```python
from build123d import *

# Parameters (mm, degrees)
IZIM1_R                     = 13.8
Y_KSEKLIK_EKSTR_ZYON1_DEPTH = 3
Y_KSEKLIK_EKSTR_ZYON2_DEPTH = 100
IZIM3_W                     = 77.5
IZIM3_H                     = 53.5
KES_EKSTR_ZYON1_DEPTH       = 10
IZIM4_W                     = 8.6
IZIM4_H                     = 8.6
KES_EKSTR_ZYON2_DEPTH       = 10
IZIM5_R                     = 1.6
KES_EKSTR_ZYON3_DEPTH       = 10
IZIM6_R                     = 1.6
KES_EKSTR_ZYON4_DEPTH       = 10
KES_EKSTR_ZYON5_START       = -10
IZIM7_R                     = 1.6
KES_EKSTR_ZYON5_DEPTH       = 10
KES_EKSTR_ZYON6_START       = -10
IZIM8_R                     = 1.6
KES_EKSTR_ZYON6_DEPTH       = 10


with BuildPart() as part:
    # Çizim1 → Yükseklik-Ekstrüzyon1 (new body)
    with BuildSketch(Plane(origin=(0, 0, 0), x_dir=(1, 0, 0), z_dir=(0, 1, 0))):
        with BuildLine():
            Line((50, 0), (140, 0))
            Line((140, 0), (140, 85))
            Line((140, 85), (0, 85))
            Line((0, 85), (0, 0))
            ThreePointArc((0, 0), (25, -25), (50, 0))
        make_face()
        with Locations(Location((25, 0, 0), (0, 0, 270))):
            Circle(IZIM1_R, mode=Mode.SUBTRACT)
    extrude(amount=Y_KSEKLIK_EKSTR_ZYON1_DEPTH)

    # Çizim2 → Yükseklik-Ekstrüzyon2 (add)
    with BuildSketch(Plane(origin=(0, 3, 0), x_dir=(1, 0, 0), z_dir=(0, 1, 0))):
        with BuildLine():
            Line((140, 85), (0, 85))
            Line((0, 85), (0, 0))
            ThreePointArc((0, 0), (25, -25), (50, 0))
            Line((50, 0), (140, 0))
            Line((140, 0), (140, 85))
        make_face()
        with BuildLine():
            Line((3, 0), (3, 3))
            Line((3, 3), (3, 82))
            Line((3, 82), (137, 82))
            Line((137, 82), (137, 3))
            Line((137, 3), (47, 3))
            Line((47, 3), (47, 0))
            ThreePointArc((47, 0), (25, -22), (3, 0))
        make_face(mode=Mode.SUBTRACT)
    extrude(amount=Y_KSEKLIK_EKSTR_ZYON2_DEPTH)

    # Çizim3 → Kes-Ekstrüzyon1 (cut)
    with BuildSketch(Plane.XY):
        with Locations((95, 66.25)):
            Rectangle(IZIM3_W, IZIM3_H)
    extrude(amount=-KES_EKSTR_ZYON1_DEPTH, mode=Mode.SUBTRACT)

    # Çizim4 → Kes-Ekstrüzyon2 (cut)
    with BuildSketch(Plane.XY):
        with Locations((95, 19.062)):
            Rectangle(IZIM4_W, IZIM4_H)
    extrude(amount=-KES_EKSTR_ZYON2_DEPTH, mode=Mode.SUBTRACT)

    # Çizim5 → Kes-Ekstrüzyon3 (cut)
    with BuildSketch(Plane.XY):
        with Locations((65, 98)):
            Circle(IZIM5_R)
        with Locations((125, 98)):
            Circle(IZIM5_R)
    extrude(amount=-KES_EKSTR_ZYON3_DEPTH, mode=Mode.SUBTRACT)

    # Çizim6 → Kes-Ekstrüzyon4 (cut)
    with BuildSketch(Plane(origin=(140, 0, 0), x_dir=(0, 0, -1), z_dir=(1, 0, 0))):
        with Locations((15, 98)):
            Circle(IZIM6_R)
        with Locations((70, 98)):
            Circle(IZIM6_R)
    extrude(amount=-KES_EKSTR_ZYON4_DEPTH, mode=Mode.SUBTRACT)

    # Çizim7 → Kes-Ekstrüzyon5 (cut)
    with BuildSketch(Plane(origin=(0, 0, -85), x_dir=(-1, 0, 0), z_dir=(0, 0, -1)).offset(KES_EKSTR_ZYON5_START)):
        with Locations(Location((-125, 98, 0), (0, 0, 180))):
            Circle(IZIM7_R)
        with Locations((-15, 98)):
            Circle(IZIM7_R)
    extrude(amount=KES_EKSTR_ZYON5_DEPTH, mode=Mode.SUBTRACT)

    # Çizim8 → Kes-Ekstrüzyon6 (cut)
    with BuildSketch(Plane.ZY.offset(KES_EKSTR_ZYON6_START)):
        with Locations(Location((-70, 98, 0), (0, 0, 180))):
            Circle(IZIM8_R)
        with Locations(Location((-15, 98, 0), (0, 0, 180))):
            Circle(IZIM8_R)
    extrude(amount=KES_EKSTR_ZYON6_DEPTH, mode=Mode.SUBTRACT)


solid = part.part
```
Work out the finished part from the listing and answer in its coordinate system (mm). A direction names the side the tool comes from. Give positions to 0.01 mm unless a question says otherwise; leave off trailing zeros. Loops run counter-clockwise (first coordinate to the right, second up) from the corner with the lowest first, then second, coordinate; pieces in that order, holes last. Notation, with made-up numbers: (-9.5, -39.75) - (22.5, -39.75) arc R31 cw to (22.5, -10.75) - close; hole circle Ø8 at (38, 57.5). An arc over 180 degrees is marked (long way). One line per question, with ' | ' between items.
(1) Straight lines are drawn through the part: probe 1 along Y at (x, z) = (125, -0.8); probe 2 along Z at (x, y) = (138, 98); probe 3 along X at (y, z) = (98, -83.45). For each, find the intervals that lie inside material, in ascending order.
Recorded:
probe 1: y = 0 to 39.5, 93 to 96.4, 99.6 to 103 | probe 2: z = -85 to -71.6, -68.4 to -16.6, -13.4 to 0 | probe 3: x = 0 to 13.4, 16.6 to 123.4, 126.6 to 140
(2) The part is cut by section C-C (y = 84). Write down the section's boundary in (x, z).
Recorded:
outline: (0, -85) - (140, -85) - (140, 0) - (133.75, 0) - (133.75, -3) - (137, -3) - (137, -82) - (3, -82) - (3, 0) arc R22 cw to (47, 0) - (47, -3) - (56.25, -3) - (56.25, 0) - (50, 0) arc R25 ccw to (0, 0) - close
(3) The part is cut by section D-D (z = -41.5). Write down the section's boundary in (x, y).
Recorded:
outline: (0, 0) - (140, 0) - (140, 103) - (137, 103) - (137, 3) - (3, 3) - (3, 103) - (0, 103) - close
(4) The part is cut by section A-A (x = 76.5). Write down the section's boundary in (y, z).
Recorded:
outline: (0, -85) - (103, -85) - (103, -82) - (3, -82) - (3, -3) - (39.5, -3) - (39.5, 0) - (0, 0) - close; (93, -3) - (103, -3) - (103, 0) - (93, 0) - close
(5) The part is cut by section B-B (y = 12). Write down the section's boundary in (x, z), then the cut area to 3 significant figures.
Recorded:
outline: (0, -85) - (140, -85) - (140, 0) - (50, 0) arc R25 ccw to (0, 0) - close; hole (3, -82) - (137, -82) - (137, -3) - (47, -3) - (47, 0) arc R22 ccw to (3, 0) - close | area: 1,400 mm²
(6) Each of these flat-tipped pins is pushed along its axis until it touches: pin 1 Ø3.5 at (x, y) = (15, 98) entering from -Z; pin 2 Ø1.9 at (y, z) = (98, -15) entering from +X; pin 3 Ø1 at (x, y) = (38, 30.5) entering from +Z. Where does it stop, or does it pass through?
Recorded:
pin 1: stops at z = -85 | pin 2: passes through | pin 3: stops at z = 21.65
(7) A tool of negligible diameter and unlimited length cuts with its end or side. For faces 1 (the face through (0, 51, -43)), 2 (the face through (16.6, 98.07, -83.48)), 3 (the face through (138.521, 98.481, -71.526)), 4 (the face through (66.526, 98.481, -1.479)), 5 (the face through (3, 52, -40)), from which of +Z, -Z, +X, -X, +Y, -Y can it reach the whole face along a straight path? Write none if from no direction.
Recorded:
face 1: +Z, -Z, -X, +Y, -Y | face 2: -Z | face 3: +X, -X | face 4: +Z | face 5: +Y
(8) The mould has two halves that part along Z. Classify faces 6 (the face through (1.52, 97.93, -13.4)), 7 (the face through (126.526, 97.519, -83.479)), 8 (the face through (24.45, 50.779, 24.994)), 9 (the face through (71, 51, -85)): +Z half, -Z half, draft (parallel to the pull), parting line (faces both ways), or undercut.
Recorded:
face 6: undercut | face 7: draft | face 8: +Z half | face 9: -Z half
